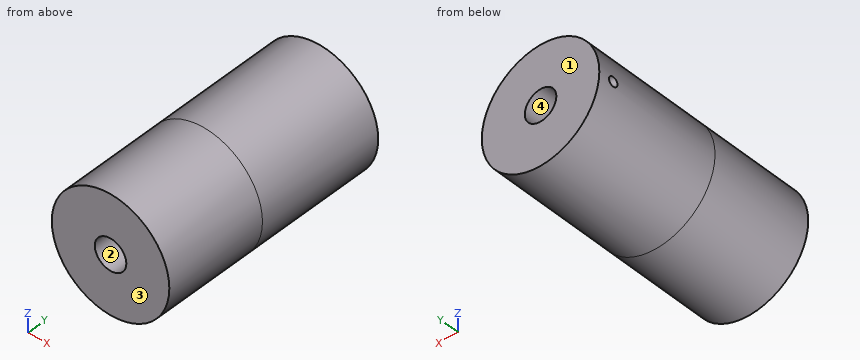
```python
from build123d import *

# Parameters (mm, degrees)
SKETCH1_R                   = 18.643111828
F_40MM_ARM_DEPTH            = 41
SKETCH2_R                   = 5
F_10MM_HOLE_10MM_DEEP_DEPTH = 10
SKETCH3_R                   = 1.5
F_0_01M_SCREW_HOLE_DEPTH    = 25
BOSS_EXTRUDE1_START         = 33
SKETCH5_R                   = 18.643111828
BOSS_EXTRUDE1_DEPTH         = 33
SKETCH4_R                   = 5
CUT_EXTRUDE2_DEPTH          = 92


with BuildPart() as part:
    # Sketch1 → 40mm arm (new body)
    with BuildSketch(Plane(origin=(0, 0, 0), x_dir=(1, 0, 0), z_dir=(0, 1, 0))):
        with Locations(Location((0, 0, 0), (0, 0, 270))):
            Circle(SKETCH1_R)
    extrude(amount=F_40MM_ARM_DEPTH)

    # Sketch2 → 10mm hole, 10mm deep (cut)
    with BuildSketch(Plane(origin=(0, 41, 0), x_dir=(1, 0, 0), z_dir=(0, 1, 0))):
        with Locations(Location((0, 0, 0), (0, 0, 270))):
            Circle(SKETCH2_R)
    extrude(amount=-F_10MM_HOLE_10MM_DEEP_DEPTH, mode=Mode.SUBTRACT)

    # Sketch3 → 0.01m screw hole (cut)
    with BuildSketch(Plane(origin=(0, 0, 0), x_dir=(0, 0, -1), z_dir=(1, 0, 0))):
        with Locations((0, 36.059550575)):
            Circle(SKETCH3_R)
    extrude(amount=-F_0_01M_SCREW_HOLE_DEPTH, mode=Mode.SUBTRACT)

    # Sketch5 → Boss-Extrude1 (add)
    with BuildSketch(Plane.XZ.offset(BOSS_EXTRUDE1_START)):
        with Locations(Location((0, 0, 0), (0, 0, 270))):
            Circle(SKETCH5_R)
    extrude(amount=-BOSS_EXTRUDE1_DEPTH)

    # Sketch4 → Cut-Extrude2 (cut)
    with BuildSketch(Plane.XZ):
        with Locations(Location((0, 0, 0), (0, 0, 90))):
            Circle(SKETCH4_R)
    extrude(amount=CUT_EXTRUDE2_DEPTH, mode=Mode.SUBTRACT)


solid = part.part
```
Could you check a few things on this model? Use its own coordinates, in mm. Face numbers are marked on the shaded views. A direction names the side the tool comes from. Round coordinates to 2 decimals unless told otherwise and drop trailing zeros. Loops run counter-clockwise (first coordinate to the right, second up) from the corner with the lowest first, then second, coordinate; pieces in that order, holes last. Notation, with made-up numbers: M -0.75,-20.75 L 28.25,-20.75 A17 cw 28.25,1.25 Z; hole C 32,64 d2. An arc over 180 degrees is marked long. Put each result on its own line as item: value.
Q1. Thinking about a two-plate mould opening in Z: for the marked faces 3 and 4, which applies, released by +Z, released by -Z, zero draft, split by the parting line, or undercut?
Check result:
face 3: zero draft
face 4: undercut
Q2. On a 3-axis mill with a long thin cutter (end or side, diameter ignored), from which of +Z, -Z, +X, -X, +Y, -Y can I reach the whole of each face in a straight line? I mean the marked faces 1 and 2. Say none if no direction works.
Check result:
face 1: +Z, -Z, +X, -X, +Y
face 2: -Y
Q3. Imagine slicing it at B-B (x = 0). Write out the boundary of the cut face in (y, z).
Check result:
outline: M -33,-18.64 L 41,-18.64 L 41,-5 L 31,-5 L 31,5 L 41,5 L 41,18.64 L -33,18.64 L -33,5 L 0,5 L 0,-5 L -33,-5 Z
Q4. For pin 1 (2 mm diameter, centred on y = -24.5, z = -12, fed in from +X); pin 2 (8 mm diameter, centred on x = -12, y = 29.5, fed in from -Z); pin 3 (3 mm diameter, centred on x = 8, y = -2, fed in from +Z), each with a flat end and sliding along its axis, tell me the tip position at first contact or that it passes through.
Check result:
pin 1: x = 15.05
pin 2: z = -16.84
pin 3: z = 17.47
Q5. Imagine slicing it at D-D (x = -7.5). Write out the boundary of the cut face in (y, z).
Check result:
outline: M -33,-17.07 L 41,-17.07 L 41,17.07 L -33,17.07 Z; hole C 36.06,0 d3
Q6. I need wall thicknesses on probe 1 along X at (y, z) = (-26, 0); probe 2 along Y at (x, z) = (-7, 0); probe 3 along X at (y, z) = (-3.5, 2). Which ranges of each line are inside material? Lowest first, please.
Check result:
probe 1: -18.64 to -5, 5 to 18.64
probe 2: -33 to 34.56, 37.56 to 41
probe 3: -18.54 to -4.58, 4.58 to 18.54
Q7. Imagine slicing it at C-C (y = 19.5). Write out the boundary of the cut face in (x, z), then the cut area to 3 significant figures.
Check result:
outline: C 0,0 d37.29
area: 1,090 mm2
Q8. Imagine slicing it at A-A (z = 0). Write out the boundary of the cut face in (x, y), then the cut area to 3 significant figures.
Check result:
outline: M -18.64,-33 L -5,-33 L -5,0 L 5,0 L 5,-33 L 18.64,-33 L 18.64,41 L 5,41 L 5,31 L -5,31 L -5,34.56 L -18.64,34.56 Z; M -18.64,37.56 L -5,37.56 L -5,41 L -18.64,41 Z
area: 2,290 mm2
